Source: CAD feature listing. Evaluate the final solid. Frame: model axes, mm. A direction names the side the tool comes from. Give positions to 0.01 mm unless a question says otherwise; leave off trailing zeros. Order: outer loops, then holes, each group sorted by start corner. A loop starts at its lowest first (then second) coordinate and runs counter-clockwise, first axis right, second up.
1) Section A-A, the plane z = -40. Return loops of the section in (x, y) (3 decimals).
2) Access query for faces 4 (the face through (35.98, 3.13, -35.75)), 5 (the face through (42.278, 3.242, 45.53)), 6 (the face through (39, 2, 48.415)), 7 (the face through (-48.415, 3, -39)), 8 (the face through (45.53, 3.242, 34.892)). Directions: +Z, -Z, +X, -X, +Y, -Y. A direction counts if a zero-diameter tool reaches every point of the face in a straight line with its end or side. Return the directions, or none.
3) Material intervals for line 1 (Z direction, x = -3.5, y = 1.25) (3 decimals); line 2 (Z direction, x = -45, y = 0.5) (3 decimals), sorted ascending.
4) Draft query along Z for faces 1 (the face through (48.415, 3, -39)), 2 (the face through (0, 3, 48.415)), 3 (the face through (0, 3, -50)). Return one class per face: released by +Z, released by -Z, zero draft, split by the parting line, or undercut.
5) First-contact query: P1, Ø0.5, axis at x = -46.5, y = 3, coming from the +Z side (3 decimals); P2, Ø2.5, axis at x = 40.755, y = 3.175, coming from the -Z side (3 decimals); P3, Ø0.9, axis at y = 4.5, z = -46, coming from the +X side (3 decimals). Flat tips, straight axial feed; report the tip coordinate or a pass-through.
6) Section B-B, the plane x = 13. Return loops of the section in (y, z) (3 decimals), plus the area to 3 significant figures.
```python
from build123d import *

# Parameters (mm, degrees)
BOSS_EXTRUDE2_DEPTH               = 6.35
FILLET7_R                         = 1.5875
FILLET8_R                         = 0.79
TAP_DRILL_FOR_4_HELICOIL5_D       = 3.048
TAP_DRILL_FOR_4_HELICOIL5_DEPTH   = 5.6896
TAP_DRILL_FOR_4_HELICOIL5_TIP     = 0.915711583
TAP_DRILL_FOR_4_HELICOIL5_2_D     = 3.048
TAP_DRILL_FOR_4_HELICOIL5_2_DEPTH = 5.6896
TAP_DRILL_FOR_4_HELICOIL5_2_TIP   = 0.915711583
FILLET10_R                        = 1.5875
TAP_DRILL_FOR_4_40_TAP1_D         = 2.2606
TAP_DRILL_FOR_4_40_TAP1_DEPTH     = 8.65
TAP_DRILL_FOR_4_40_TAP1_TIP       = 0.679152758
CHAMFER1_SIZE                     = 17
FILLET11_R                        = 1.5875
TAP_DRILL_FOR_4_HELICOIL6_D       = 3.048
TAP_DRILL_FOR_4_HELICOIL6_DEPTH   = 5.6896
TAP_DRILL_FOR_4_HELICOIL6_TIP     = 0.915711583
TAP_DRILL_FOR_4_HELICOIL7_D       = 3.048
TAP_DRILL_FOR_4_HELICOIL7_DEPTH   = 5.69
TAP_DRILL_FOR_4_HELICOIL7_TIP     = 0.915711583


with BuildPart() as part:
    # Sketch10 → Boss-Extrude2 (new body)
    with BuildSketch(Plane(origin=(0, 0, 0), x_dir=(1, 0, 0), z_dir=(0, 1, 0))):
        Polygon((48.415, -48.415), (29.365, -48.415), (29.365, -50), (-29.365, -50), (-29.365, -48.415), (-48.415, -48.415), (-48.415, -29.365), (-50, -29.365), (-50, 29.365), (-48.415, 29.365), (-48.415, 48.415), (-29.365, 48.415), (-29.365, 50), (29.365, 50), (29.365, 48.415), (48.415, 48.415), (48.415, 29.365), (50, 29.365), (50, -29.365), (48.415, -29.365), align=None)
        Polygon((27.365, 48.415), (-27.365, 48.415), (-27.365, 46.415), (-27.365, 27.365), (-46.415, 27.365), (-48.415, 27.365), (-48.415, -27.365), (-46.415, -27.365), (-27.365, -27.365), (-27.365, -46.415), (-27.365, -48.415), (27.365, -48.415), (27.365, -46.415), (27.365, -27.365), (46.415, -27.365), (48.415, -27.365), (48.415, 27.365), (46.415, 27.365), (27.365, 27.365), (27.365, 46.415), align=None, mode=Mode.SUBTRACT)
    extrude(amount=BOSS_EXTRUDE2_DEPTH)

    # Fillet7
    # the kernel refuses this fillet: 1.5875 mm, written as the material it adds along each edge
    with BuildSketch(Plane(origin=(-48.415, 0, 29.365), x_dir=(-1, 0, 0), z_dir=(0, 1, 0))) as fillet7_piece_1_section:
        with BuildLine():
            CenterArc((FILLET7_R, FILLET7_R), FILLET7_R, 180, 90)
            Line((0, FILLET7_R), (0, 0))
            Line((0, 0), (FILLET7_R, 0))
        make_face()
    fillet7_piece_1 = extrude(amount=6.35, mode=Mode.PRIVATE)
    fillet7_piece_1 = split(fillet7_piece_1, bisect_by=Plane(origin=(-50, 3.175, 29.724448602), z_dir=(1, 0, 0)), keep=Keep.TOP, mode=Mode.PRIVATE)
    add(fillet7_piece_1)
    with BuildSketch(Plane(origin=(-29.365, 0, 48.415), x_dir=(-1, 0, 0), z_dir=(0, 1, 0))) as fillet7_piece_2_section:
        with BuildLine():
            CenterArc((FILLET7_R, FILLET7_R), FILLET7_R, 180, 90)
            Line((0, FILLET7_R), (0, 0))
            Line((0, 0), (FILLET7_R, 0))
        make_face()
    fillet7_piece_2 = extrude(amount=6.35, mode=Mode.PRIVATE)
    fillet7_piece_2 = split(fillet7_piece_2, bisect_by=Plane(origin=(-29.724448602, 3.175, 50), z_dir=(0, 0, -1)), keep=Keep.TOP, mode=Mode.PRIVATE)
    add(fillet7_piece_2)
    with BuildSketch(Plane(origin=(29.365, 0, 48.415), x_dir=(1, 0, 0), z_dir=(0, 1, 0))) as fillet7_piece_3_section:
        with BuildLine():
            CenterArc((FILLET7_R, -FILLET7_R), FILLET7_R, 90, 90)
            Line((0, -FILLET7_R), (0, 0))
            Line((0, 0), (FILLET7_R, 0))
        make_face()
    fillet7_piece_3 = extrude(amount=6.35, mode=Mode.PRIVATE)
    fillet7_piece_3 = split(fillet7_piece_3, bisect_by=Plane(origin=(29.724448602, 3.175, 50), z_dir=(0, 0, -1)), keep=Keep.TOP, mode=Mode.PRIVATE)
    add(fillet7_piece_3)
    with BuildSketch(Plane(origin=(48.415, 0, 29.365), x_dir=(1, 0, 0), z_dir=(0, 1, 0))) as fillet7_piece_4_section:
        with BuildLine():
            CenterArc((FILLET7_R, -FILLET7_R), FILLET7_R, 90, 90)
            Line((0, -FILLET7_R), (0, 0))
            Line((0, 0), (FILLET7_R, 0))
        make_face()
    fillet7_piece_4 = extrude(amount=6.35, mode=Mode.PRIVATE)
    fillet7_piece_4 = split(fillet7_piece_4, bisect_by=Plane(origin=(50, 3.175, 29.724448602), z_dir=(-1, 0, 0)), keep=Keep.TOP, mode=Mode.PRIVATE)
    add(fillet7_piece_4)
    with BuildSketch(Plane(origin=(48.415, 0, -29.365), x_dir=(1, 0, 0), z_dir=(0, 1, 0))) as fillet7_piece_5_section:
        with BuildLine():
            CenterArc((FILLET7_R, FILLET7_R), FILLET7_R, 180, 90)
            Line((0, FILLET7_R), (0, 0))
            Line((0, 0), (FILLET7_R, 0))
        make_face()
    fillet7_piece_5 = extrude(amount=6.35, mode=Mode.PRIVATE)
    fillet7_piece_5 = split(fillet7_piece_5, bisect_by=Plane(origin=(50, 3.175, -29.724448602), z_dir=(-1, 0, 0)), keep=Keep.TOP, mode=Mode.PRIVATE)
    add(fillet7_piece_5)
    with BuildSketch(Plane(origin=(29.365, 0, -48.415), x_dir=(1, 0, 0), z_dir=(0, 1, 0))) as fillet7_piece_6_section:
        with BuildLine():
            CenterArc((FILLET7_R, FILLET7_R), FILLET7_R, 180, 90)
            Line((0, FILLET7_R), (0, 0))
            Line((0, 0), (FILLET7_R, 0))
        make_face()
    fillet7_piece_6 = extrude(amount=6.35, mode=Mode.PRIVATE)
    fillet7_piece_6 = split(fillet7_piece_6, bisect_by=Plane(origin=(29.724448602, 3.175, -50), z_dir=(0, 0, 1)), keep=Keep.TOP, mode=Mode.PRIVATE)
    add(fillet7_piece_6)
    with BuildSketch(Plane(origin=(-48.415, 0, -29.365), x_dir=(0, 0, -1), z_dir=(0, 1, 0))) as fillet7_piece_7_section:
        with BuildLine():
            CenterArc((FILLET7_R, FILLET7_R), FILLET7_R, 180, 90)
            Line((0, FILLET7_R), (0, 0))
            Line((0, 0), (FILLET7_R, 0))
        make_face()
    fillet7_piece_7 = extrude(amount=6.35, mode=Mode.PRIVATE)
    fillet7_piece_7 = split(fillet7_piece_7, bisect_by=Plane(origin=(-50, 3.175, -29.724448602), z_dir=(1, 0, 0)), keep=Keep.TOP, mode=Mode.PRIVATE)
    add(fillet7_piece_7)
    with BuildSketch(Plane(origin=(-29.365, 0, -48.415), x_dir=(0, 0, -1), z_dir=(0, 1, 0))) as fillet7_piece_8_section:
        with BuildLine():
            CenterArc((FILLET7_R, FILLET7_R), FILLET7_R, 180, 90)
            Line((0, FILLET7_R), (0, 0))
            Line((0, 0), (FILLET7_R, 0))
        make_face()
    fillet7_piece_8 = extrude(amount=6.35, mode=Mode.PRIVATE)
    fillet7_piece_8 = split(fillet7_piece_8, bisect_by=Plane(origin=(-29.724448602, 3.175, -50), z_dir=(0, 0, 1)), keep=Keep.TOP, mode=Mode.PRIVATE)
    add(fillet7_piece_8)

    # Fillet8
    fillet8_edges = [part.edges().sort_by_distance(p)[0] for p in [
        (-48.415, 3.175, -48.415),
        (48.415, 3.175, -48.415),
        (48.415, 3.175, 48.415),
        (-48.415, 3.175, 48.415),
    ]]
    fillet(fillet8_edges, radius=FILLET8_R)

    # Tap Drill for _4 Helicoil5
    with Locations(Plane(origin=(48.415, 0, 0), x_dir=(0, 0, -1), z_dir=(1, 0, 0))):
        with Locations((-36.415, 3.175), (36.415, 3.175)):
            Hole(TAP_DRILL_FOR_4_HELICOIL5_D / 2, depth=TAP_DRILL_FOR_4_HELICOIL5_DEPTH)
            with Locations((0, 0, -(TAP_DRILL_FOR_4_HELICOIL5_DEPTH + TAP_DRILL_FOR_4_HELICOIL5_TIP / 2))):  # 118° drill point
                Cone(0, TAP_DRILL_FOR_4_HELICOIL5_D / 2, TAP_DRILL_FOR_4_HELICOIL5_TIP, mode=Mode.SUBTRACT)

    # Tap Drill for _4 Helicoil5 2
    with Locations(Plane.XY.offset(48.415)):
        with Locations((40.755, 3.175), (-41.615, 3.175)):
            Hole(TAP_DRILL_FOR_4_HELICOIL5_2_D / 2, depth=TAP_DRILL_FOR_4_HELICOIL5_2_DEPTH)
            with Locations((0, 0, -(TAP_DRILL_FOR_4_HELICOIL5_2_DEPTH + TAP_DRILL_FOR_4_HELICOIL5_2_TIP / 2))):  # 118° drill point
                Cone(0, TAP_DRILL_FOR_4_HELICOIL5_2_D / 2, TAP_DRILL_FOR_4_HELICOIL5_2_TIP, mode=Mode.SUBTRACT)

    # Fillet10
    fillet10_edges = [part.edges().sort_by_distance(p)[0] for p in [
        (27.365, 3.175, -48.415),
        (-27.365, 3.175, -48.415),
        (-48.415, 3.175, -27.365),
        (-48.415, 3.175, 27.365),
        (-27.365, 3.175, 48.415),
        (27.365, 3.175, 48.415),
        (48.415, 3.175, 27.365),
        (48.415, 3.175, -27.365),
    ]]
    fillet(fillet10_edges, radius=FILLET10_R)

    # Tap Drill for #4-40 Tap1
    with Locations(Plane(origin=(0, 6.35, 0), x_dir=(1, 0, 0), z_dir=(0, 1, 0))):
        with Locations((37.465, -42.8625), (40.005, 42.8625), (-40.005, 42.8625), (-36.195, -42.8625)):
            Hole(TAP_DRILL_FOR_4_40_TAP1_D / 2, depth=TAP_DRILL_FOR_4_40_TAP1_DEPTH)
            with Locations((0, 0, -(TAP_DRILL_FOR_4_40_TAP1_DEPTH + TAP_DRILL_FOR_4_40_TAP1_TIP / 2))):  # 118° drill point
                Cone(0, TAP_DRILL_FOR_4_40_TAP1_D / 2, TAP_DRILL_FOR_4_40_TAP1_TIP, mode=Mode.SUBTRACT)

    # Chamfer1
    chamfer1_edges = [part.edges().sort_by_distance(p)[0] for p in [
        (27.365, 3.175, -27.365),
        (-27.365, 3.175, -27.365),
        (-27.365, 3.175, 27.365),
        (27.365, 3.175, 27.365),
    ]]
    chamfer(chamfer1_edges, length=CHAMFER1_SIZE)

    # Fillet11
    fillet11_edges = [part.edges().sort_by_distance(p)[0] for p in [
        (-44.365, 3.175, 27.365),
        (-27.365, 3.175, 44.365),
        (27.365, 3.175, 44.365),
        (44.365, 3.175, 27.365),
        (-27.365, 3.175, -44.365),
        (-44.365, 3.175, -27.365),
        (44.365, 3.175, -27.365),
        (27.365, 3.175, -44.365),
    ]]
    fillet(fillet11_edges, radius=FILLET11_R)

    # Tap Drill for #4 Helicoil6
    with Locations(Plane(origin=(0, 0, -48.415), x_dir=(-1, 0, 0), z_dir=(0, 0, -1))):
        with Locations((36.415, 3.175), (-36.415, 3.175)):
            Hole(TAP_DRILL_FOR_4_HELICOIL6_D / 2, depth=TAP_DRILL_FOR_4_HELICOIL6_DEPTH)
            with Locations((0, 0, -(TAP_DRILL_FOR_4_HELICOIL6_DEPTH + TAP_DRILL_FOR_4_HELICOIL6_TIP / 2))):  # 118° drill point
                Cone(0, TAP_DRILL_FOR_4_HELICOIL6_D / 2, TAP_DRILL_FOR_4_HELICOIL6_TIP, mode=Mode.SUBTRACT)

    # Tap Drill for #4 Helicoil7
    with Locations(Plane.ZY.offset(48.415)):
        with Locations((-36.415, 3.175), (36.415, 3.175)):
            Hole(TAP_DRILL_FOR_4_HELICOIL7_D / 2, depth=TAP_DRILL_FOR_4_HELICOIL7_DEPTH)
            with Locations((0, 0, -(TAP_DRILL_FOR_4_HELICOIL7_DEPTH + TAP_DRILL_FOR_4_HELICOIL7_TIP / 2))):  # 118° drill point
                Cone(0, TAP_DRILL_FOR_4_HELICOIL7_D / 2, TAP_DRILL_FOR_4_HELICOIL7_TIP, mode=Mode.SUBTRACT)


solid = part.part
```
From the geometry:
1. outline: (-48.415, 0) - (-31.73, 0) - (-31.73, 6.35) - (-48.415, 6.35) - close; (31.73, 0) - (48.415, 0) - (48.415, 6.35) - (31.73, 6.35) - close
2. face 4: +Y, -Y
2. face 5: +Z
2. face 6: +Z, +X, +Y, -Y
2. face 7: -Z, -X, +Y, -Y
2. face 8: +X
3. line 1: z = -50 to -48.415, 48.415 to 50
3. line 2: z = -48.415 to -27.365, 27.365 to 48.415
4. face 1: zero draft
4. face 2: undercut
4. face 3: released by -Z
5. P1: stops at z = 48.415
5. P2: stops at z = -48.415
5. P3: stops at x = 48.415
6. outline: (0, -50) - (6.35, -50) - (6.35, -48.415) - (0, -48.415) - close; (0, 48.415) - (6.35, 48.415) - (6.35, 50) - (0, 50) - close
6. area: 20.1 mm2
